Input: part model. Units: mm. Frame: model coordinates. A direction names the side the tool comes from. Coordinates: 2 decimals unless noted, no trailing zeros. Write each loop counter-clockwise with the first axis right and the second up, starting at its lowest first coordinate (ties: lowest second). Pieces come first, ordered by that corner, then holes. Notation, with made-up numbers: (21, 12) - (38, 12) arc R21 cw to (38, 30) - close; hole circle Ø1 at (79.25, -23). An arc over 180 degrees is marked (long way). Put each result on its own line as item: value. Start each with the question number.
1. Cut plane B-B, the plane y = -8.5. Return loops of the section in (x, z).
2. Cut plane C-C, the plane z = 7. Return loops of the section in (x, y).
3. Pull-direction query (X, two-part tool) for faces 1 (the cylindrical face through (-37.15, 0.08, 2.46)), 2 (the flat face through (-1, 0, 5)), 3 (the flat face through (52.5, 0, 24)); classes: released by +X, released by -X, zero draft, split by the parting line, or undercut.
4. Cut plane D-D, the plane x = -38.5. Return loops of the section in (y, z), and give its area (3 significant figures).
5. Access query for faces 4 (the flat face through (47.5, -0.3, 22.3)), 5 (the flat face through (50, 0, 40)). Directions: +Z, -Z, +X, -X, +Y, -Y. A direction counts if a zero-diameter tool reaches every point of the face in a straight line with its end or side. Return the directions, or none.
6. Pin query (flat end, axial travel): pin 1 (3 mm diameter, centred on x = -20.9, y = 0, fed in from -Z); pin 2 (12.5 mm diameter, centred on x = -8, y = 9, fed in from +Z). Return the tip coordinate at first contact, or that it passes through.
7. Cut plane A-A, the plane x = -20.9. Return loops of the section in (y, z), and give its area (4 significant figures).
8. Line query: line 1 (X direction, y = 7.5, z = 37.5); line 2 (Z direction, x = 25, y = 0); line 3 (Y direction, x = 51.3, z = 20) (3 decimals). Output: solid intervals per line, ascending.
from build123d import *

# Parameters (mm, degrees)
F0_W     = 5
F0_H     = 42
F1_DEPTH = 40
F2_DEPTH = 5
F4_DEPTH = 5


with BuildPart() as f1:
    # F0 (on Top) → F1 (new body)
    with BuildSketch(Plane.XY):
        with Locations((50, 0)):
            Rectangle(F0_W, F0_H)
    extrude(amount=F1_DEPTH)

    # F0 (on Top) → F2 (join)
    with BuildSketch(Plane.XY):
        Polygon((47.5, 21), (-47.5, 21), (-47.5, 0), (-47.5, -21), (47.5, -21), align=None)
        with BuildLine():
            ThreePointArc((-37.15, 0), (-38.9, -1.75), (-40.65, 0))
            ThreePointArc((-40.65, 0), (-38.9, 1.75), (-37.15, 0))
        make_face(mode=Mode.SUBTRACT)
        with BuildLine():
            ThreePointArc((-19.15, 0), (-20.9, -1.75), (-22.65, 0))
            ThreePointArc((-22.65, 0), (-20.9, 1.75), (-19.15, 0))
        make_face(mode=Mode.SUBTRACT)
    extrude(amount=F2_DEPTH)

    # F3 (on face) → F4 (cut)
    with BuildSketch(Plane.YZ.offset(52.5)):
        with BuildLine():
            ThreePointArc((1.925, 20), (-1.361181, 21.361181), (0, 18.075))
            ThreePointArc((0, 18.075), (1.361181, 18.638819), (1.925, 20))
        make_face()
    extrude(amount=-F4_DEPTH, mode=Mode.SUBTRACT)


solid = f1.part
Report:
1. outline: (-47.5, 0) - (52.5, 0) - (52.5, 40) - (47.5, 40) - (47.5, 5) - (-47.5, 5) - close
2. outline: (47.5, -21) - (52.5, -21) - (52.5, 21) - (47.5, 21) - close
3. face 1: undercut
3. face 2: zero draft
3. face 3: released by +X
4. outline: (-21, 0) - (-1.7, 0) - (-1.7, 5) - (-21, 5) - close; (1.7, 0) - (21, 0) - (21, 5) - (1.7, 5) - close
4. area: 193 mm^2
5. face 4: +Z, -X, +Y, -Y
5. face 5: +Z, +X, -X, +Y, -Y
6. pin 1: passes through
6. pin 2: stops at z = 5
7. outline: (-21, 0) - (-1.75, 0) - (-1.75, 5) - (-21, 5) - close; (1.75, 0) - (21, 0) - (21, 5) - (1.75, 5) - close
7. area: 192.5 mm^2
8. line 1: x = 47.5 to 52.5
8. line 2: z = 0 to 5
8. line 3: y = -21 to -1.925, 1.925 to 21
